Input: part model. Units: mm. Frame: model coordinates. A direction names the side the tool comes from. Give positions to 0.01 mm unless a question says otherwise; leave off trailing zeros. Loops run counter-clockwise (first coordinate to the right, second up) from the corner with the lowest first, then second, coordinate; pieces in that order, holes last. Notation, with made-up numbers: M 79,50.25 L 90,50.25 A14 cw 90,56.25 Z; hole C -32.75,50.5 d2. An arc over 180 degrees is marked long. Answer as a JSON object with one key per item and string values. Group by question number.
1) Access query for faces 1 (the flat face through (-2, -1, -14.8)), 2 (the cylindrical face through (-11.18, 1.6, 3.71)), 3 (the flat face through (-10.622, 11, 5)). Directions: +Z, -Z, +X, -X, +Y, -Y. A direction counts if a zero-diameter tool reaches every point of the face in a straight line with its end or side. Return the directions, or none.
2) Section query A-A on z = 1. Return loops of the section in (x, y), plus the area to 3 significant figures.
3) Section query B-B on z = -2.8. Return loops of the section in (x, y).
4) First-contact query: P1, Ø3, axis at x = -7, z = -4, coming from the +Y side; P2, Ø1.4, axis at x = -2.07, z = -2.8, coming from the -Y side; P3, Ø1.6, axis at y = -1, z = -7.5, coming from the -X side; P4, Ø0.7, axis at x = -9.5, y = 2, coming from the -Z side. Flat tips, straight axial feed; report the tip coordinate or a pass-through.
5) Ray query, L1, parallel to Y at x = -5.5, z = 2.5; L2, parallel to X at y = 11.75, z = 2.5; L3, parallel to Z at x = -7.75, y = 23.75. Return the intervals inside material, ascending.
6) Section query C-C on y = 17.51. Return loops of the section in (x, z), plus the area to 3 significant figures.
7) Draft query along Z for faces 4 (the cylindrical face through (-3.024, -1.014, -3.53)), 5 (the flat face through (7.478, 12, 2)), 6 (the flat face through (-10, 2, -0.8)). Return one class per face: +Z half, -Z half, draft (parallel to the pull), parting line (faces both ways), or undercut.
8) Section query D-D on x = -1.25. Return loops of the section in (y, z).
from build123d import *

# Parameters (mm, degrees)
F0_W      = 23.1
F0_H      = 27.7
F1_DEPTH  = 5.2
F2_W      = 19.1
F2_H      = 23.7
F3_DEPTH  = 4.2
F4_R      = 1.4
F4_R_2    = 1.2
F5_DEPTH  = 1
F6_R      = 1
F7_DEPTH  = 4
F8_W      = 23.1
F8_H      = 27.7
F8_R      = 1.2
F9_DEPTH  = 6.001
F10_R     = 2
F11_W     = 7
F11_H     = 20
F11_R     = 1.2
F12_DEPTH = 2


with BuildPart() as f1:
    # F0 (on Top) → F1 (new body)
    with BuildSketch(Plane.XY):
        with Locations((-2.071892, 11.85)):
            Rectangle(F0_W, F0_H)
        with BuildLine():
            Line((-10.621892, 8.53), (-10.621892, 13.53))
            ThreePointArc((-10.621892, 13.53), (-9.596766, 16.004874), (-7.121892, 17.03))
            ThreePointArc((-7.121892, 17.03), (-4.647019, 16.004874), (-3.621892, 13.53))
            Line((-3.621892, 13.53), (-3.621892, 8.53))
            ThreePointArc((-3.621892, 8.53), (-4.647019, 6.055126), (-7.121892, 5.03))
            ThreePointArc((-7.121892, 5.03), (-9.596766, 6.055126), (-10.621892, 8.53))
        make_face(mode=Mode.SUBTRACT)
    extrude(amount=F1_DEPTH)

    # F2 (on Top) → F3 (cut)
    with BuildSketch(Plane.XY):
        with Locations((-2.071892, 11.85)):
            Rectangle(F2_W, F2_H)
    extrude(amount=F3_DEPTH, mode=Mode.SUBTRACT)

    # F4 (on face) → F5 (join)
    with BuildSketch(Plane(origin=(0, 0, 4.2), x_dir=(1, 0, 0), z_dir=(0, 0, -1))):
        with Locations((5.508108, -17.51)):
            Circle(F4_R)
        with Locations((-9.981892, -1.65)):
            Circle(F4_R_2)
    extrude(amount=F5_DEPTH)

    # F6 (on face) → F7 (join)
    with BuildSketch(Plane(origin=(0, 0, 3.2), x_dir=(1, 0, 0), z_dir=(0, 0, -1))):
        with Locations((-9.981892, -1.65)):
            Circle(F6_R)
        with Locations((5.508108, -17.51)):
            Circle(F6_R)
    extrude(amount=F7_DEPTH)

    # F8 (on face) → F9 (intersect, through all)
    with BuildSketch(Plane.XY.offset(5.2)):
        with Locations((-2.071892, 11.85)):
            Rectangle(F8_W, F8_H)
        with Locations((-10.169229, 4.364627)):
            Circle(F8_R, mode=Mode.SUBTRACT)
        with BuildLine():
            Line((-3.621892, 13.53), (-3.621892, 8.53))
            ThreePointArc((-3.621892, 8.53), (-7.121892, 5.03), (-10.621892, 8.53))
            Line((-10.621892, 8.53), (-10.621892, 13.53))
            ThreePointArc((-10.621892, 13.53), (-7.121892, 17.03), (-3.621892, 13.53))
        make_face(mode=Mode.SUBTRACT)
    extrude(amount=-F9_DEPTH, mode=Mode.INTERSECT)

    # F10
    f10_edges = [f1.edges().sort_by_distance(p)[0] for p in [
        (-13.621892, 25.7, 2.6),
        (-13.621892, -2, 2.6),
        (9.478108, -2, 2.6),
        (9.478108, 25.7, 2.6),
    ]]
    fillet(f10_edges, radius=F10_R)

    # F11 (on face) → F12 (join)
    with BuildSketch(Plane.XZ.offset(2)):
        with Locations((-2.071892, -4.8)):
            Rectangle(F11_W, F11_H)
        with Locations((-2.071892, -7.2)):
            Circle(F11_R, mode=Mode.SUBTRACT)
        with Locations((-2.071892, -11.6)):
            Circle(F11_R, mode=Mode.SUBTRACT)
        with Locations((-2.071892, -2.8)):
            Circle(F11_R, mode=Mode.SUBTRACT)
    extrude(amount=-F12_DEPTH)


solid = f1.part
Output:
{
 "1": {"face 1": "-Z, +X, -X, +Y, -Y", "face 2": "-Z", "face 3": "+Z, -Z"},
 "2": {"outline": "M -13.62,0 A2 ccw -11.62,-2 L 7.48,-2 A2 ccw 9.48,0 L 9.48,23.7 A2 ccw 7.48,25.7 L -11.62,25.7 A2 ccw -13.62,23.7 Z; C -9.98,1.65 d2; C 5.51,17.51 d2; hole M -11.62,0 L 7.48,0 L 7.48,23.7 L -11.62,23.7 Z", "area": "190 mm^2"},
 "3": {"outline": "M -5.57,-2 L -3.27,-2 L -3.27,0 L -5.57,0 Z; M -0.87,-2 L 1.43,-2 L 1.43,0 L -0.87,0 Z"},
 "4": {"P1": "stops at y = 0", "P2": "passes through", "P3": "stops at x = -5.57", "P4": "stops at z = -0.8"},
 "5": {"L1": "y = -2 to 0, 23.7 to 25.7", "L2": "x = -13.62 to -11.62, 7.48 to 9.48", "L3": "z = 0 to 5.2"},
 "6": {"outline": "M -13.62,0 L -11.62,0 L -11.62,4.2 L 4.11,4.2 L 4.11,3.2 L 4.51,3.2 L 4.51,-0.8 L 6.51,-0.8 L 6.51,3.2 L 6.91,3.2 L 6.91,4.2 L 7.48,4.2 L 7.48,0 L 9.48,0 L 9.48,5.2 L -13.62,5.2 Z", "area": "50.7 mm^2"},
 "7": {"face 4": "undercut", "face 5": "draft", "face 6": "-Z half"},
 "8": {"outline": "M -2,-14.8 L 0,-14.8 L 0,-12.47 L -2,-12.47 Z; M -2,-10.73 L 0,-10.73 L 0,-8.07 L -2,-8.07 Z; M -2,-6.33 L 0,-6.33 L 0,-3.67 L -2,-3.67 Z; M -2,-1.93 L 0,-1.93 L 0,4.2 L 23.7,4.2 L 23.7,0 L 25.7,0 L 25.7,5.2 L -2,5.2 Z"}
}
